Input: part model. Units: mm. Frame: model coordinates. Give positions to 0.01 mm unless a question says otherwise; leave off trailing zeros. Write each loop counter-clockwise with the first axis right and the second up, starting at its lowest first coordinate (ties: lowest second). Pieces come first, ordered by that corner, then holes.
```python
from build123d import *

# Parameters (mm, degrees)
SKETCH1_R           = 38.1
SKETCH1_R_2         = 36.1
BOSS_EXTRUDE1_DEPTH = 457.2
SKETCH2_W           = 3.81
SKETCH2_H           = 25.4
CUT_EXTRUDE1_DEPTH  = 39.1
CIRPATTERN1_COUNT   = 3


with BuildPart() as part:
    # Sketch1 → Boss-Extrude1 (new body)
    with BuildSketch(Plane(origin=(0, 0, 0), x_dir=(1, 0, 0), z_dir=(0, 1, 0))):
        Circle(SKETCH1_R)
        Circle(SKETCH1_R_2, mode=Mode.SUBTRACT)
    extrude(amount=BOSS_EXTRUDE1_DEPTH)

    # Sketch2 → Cut-Extrude1 (cut, through all)
    with BuildSketch(Plane.XY):
        with Locations((0, 38.1)):
            Rectangle(SKETCH2_W, SKETCH2_H)
    cut_extrude1 = extrude(amount=-CUT_EXTRUDE1_DEPTH, mode=Mode.SUBTRACT)

    # CirPattern1: Cut-Extrude1 ×3 about axis
    cirpattern1_axis = Axis((0, 0, 0), (0, 1, 0))
    for i in range(1, CIRPATTERN1_COUNT):
        add(cut_extrude1.rotate(cirpattern1_axis, i * 360 / CIRPATTERN1_COUNT), mode=Mode.SUBTRACT)


solid = part.part
```
Item 1: Ray query, line 1 (X direction, y = 169, z = 0); line 2 (X direction, y = 324, z = 17.5). Return the intervals inside material, ascending.
Item 2: Section B-B (x = -15). Return loops of the section in (y, z).
Item 3: Section C-C (y = 102.5). Return loops of the section in (x, z), and give its area (3 significant figures).
Item 4: Mould query, pull axis X, two halves, no side actions, for faces 1 (the cylindrical face through (-30.235, 225.4, 23.183)), 2 (the cylindrical face through (-7.83, 225.4, 35.24)), 3 (the flat face through (14, 457.2, 34)). Classes: +X half, -X half, draft (parallel to the pull), parting line (faces both ways), or undercut.
Item 5: Pin query (flat end, axial travel): pin 1 (1.5 mm diameter, centred on y = 249.5, z = 16, fed in from -X); pin 2 (3 mm diameter, centred on y = 329, z = 27, fed in from +X); pin 3 (2 mm diameter, centred on y = 76, z = 14, fed in from +X). Return the tip coordinate at first contact, or that it passes through.
Item 6: Section A-A (z = 0). Return loops of the section in (x, y), and give its area (3 significant figures).
Solved:
1. line 1: x = -38.1 to -36.1, 36.1 to 38.1
1. line 2: x = -33.84 to -31.57, 31.57 to 33.84
2. outline: (0, -35.02) - (457.2, -35.02) - (457.2, -32.84) - (0, -32.84) - close; (0, 32.84) - (457.2, 32.84) - (457.2, 35.02) - (0, 35.02) - close
3. outline: circle Ø76.2 at (0, 0); hole circle Ø72.2 at (0, 0)
3. area: 466 mm2
4. face 1: parting line
4. face 2: undercut
4. face 3: draft
5. pin 1: stops at x = -34.91
5. pin 2: stops at x = 28.31
5. pin 3: stops at x = 35.81
6. outline: (-38.1, 0) - (-36.1, 0) - (-36.1, 457.2) - (-38.1, 457.2) - close; (36.1, 0) - (38.1, 0) - (38.1, 457.2) - (36.1, 457.2) - close
6. area: 1,830 mm2
